The listing builds one solid part. Answer for the finished solid, in the listing's coordinates (mm). A direction names the side the tool comes from. Give positions to 0.01 mm unless a question says otherwise; leave off trailing zeros. Order: outer loops, then holes, each group sorted by start corner. A loop starts at its lowest first (then second) coordinate and runs counter-clockwise, first axis right, second up.
```python
from build123d import *

# Parameters (mm, degrees)
DIAM_TRE_DU_PER_AGE_4_0_4_1_D     = 4
DIAM_TRE_DU_PER_AGE_4_0_4_1_DEPTH = 5
DIAM_TRE_DU_PER_AGE_4_0_4_1_TIP   = 1.201721238
TROU_TARAUD_M41_D                 = 3.3
R_P_TITION_CIRCULAIRE1_COUNT      = 4
CHANFREIN1_SIZE                   = 0.5


with BuildPart() as part:
    # Esquisse1 → Révolution1 (revolve)
    with BuildSketch(Plane(origin=(0, 0, 0), x_dir=(0, 0, -1), z_dir=(1, 0, 0))):
        Polygon((-31, -3), (-31, 0), (-32.5, 0), (-32.5, 7), (-42, 7), (-42, -3), align=None)
    revolve(axis=Axis((0, 0, 0), (0, -1, 0)))

    # Diamètre du perçage Ø4.0 (4)1
    with Locations(Plane(origin=(0, 7, 0), x_dir=(1, 0, 0), z_dir=(0, 1, 0))):
        with Locations((0, 37), (0, -37)):
            Hole(DIAM_TRE_DU_PER_AGE_4_0_4_1_D / 2, depth=DIAM_TRE_DU_PER_AGE_4_0_4_1_DEPTH)
            with Locations((0, 0, -(DIAM_TRE_DU_PER_AGE_4_0_4_1_DEPTH + DIAM_TRE_DU_PER_AGE_4_0_4_1_TIP / 2))):  # 118° drill point
                Cone(0, DIAM_TRE_DU_PER_AGE_4_0_4_1_D / 2, DIAM_TRE_DU_PER_AGE_4_0_4_1_TIP, mode=Mode.SUBTRACT)

    # Trou taraudé M41 (through all)
    with Locations(Plane(origin=(0, 7, 0), x_dir=(1, 0, 0), z_dir=(0, 1, 0))):
        with Locations((-26.162950904, 26.162950904)):
            trou_taraud_m41 = Hole(TROU_TARAUD_M41_D / 2)

    # Répétition circulaire1: Trou taraudé M41 ×4 about axis
    r_p_tition_circulaire1_axis = Axis((0, 0, 0), (0, 1, 0))
    for i in range(1, R_P_TITION_CIRCULAIRE1_COUNT):
        add(trou_taraud_m41.rotate(r_p_tition_circulaire1_axis, i * 360 / R_P_TITION_CIRCULAIRE1_COUNT), mode=Mode.SUBTRACT)

    # Chanfrein1
    chanfrein1_edges = [part.edges().sort_by_distance(p)[0] for p in [
        (0, 7, -32.5),
    ]]
    chamfer(chanfrein1_edges, length=CHANFREIN1_SIZE)


solid = part.part
```
1) Given P1, Ø4, axis at x = 26.16, z = -26.16, coming from the +Y side; P2, Ø3, axis at x = -21, y = 2.5, coming from the +Z side; P3, Ø3, axis at y = 1.5, z = -18, coming from the +X side; P4, Ø5, axis at x = 13, y = 5.5, coming from the -Z side, each flat-ended and moving along its own axis, determine where each tip first touches the part or whether it passes through.
Geometry says:
P1: stops at y = 7
P2: stops at z = 37.2
P3: stops at x = 38.62
P4: stops at z = -40.67
2) A tool of negligible diameter and unlimited length cuts with its end or side. For faces 4 (the flat face through (12, 0, -29)), 5 (the cylindrical face through (-27.687, 1.93, -25.531)), from which of +Z, -Z, +X, -X, +Y, -Y can it reach the whole face along a straight path? Write none if from no direction.
Geometry says:
face 4: +Y
face 5: +Y, -Y
3) Find section A-A (z = 0). Write down the section's boundary in (x, y), then the cut area to 3 significant figures.
Geometry says:
outline: (-42, -3) - (-31, -3) - (-31, 0) - (-32.5, 0) - (-32.5, 6.5) - (-33, 7) - (-42, 7) - close; (31, -3) - (42, -3) - (42, 7) - (33, 7) - (32.5, 6.5) - (32.5, 0) - (31, 0) - close
area: 199 mm2
4) Straight lines are drawn through the part: probe 1 along Z at (x, y) = (0, 5.1); probe 2 along Z at (x, y) = (13, 6.25); probe 3 along X at (y, z) = (-0.75, -12). For each, find the intervals that lie inside material, in ascending order.
Geometry says:
probe 1: z = -42 to -39, -35 to -32.5, 32.5 to 35, 39 to 42
probe 2: z = -39.94 to -29.79, 29.79 to 39.94
probe 3: x = -40.25 to -28.58, 28.58 to 40.25
5) For a pull along X with two mould halves and no side action, classify faces 1 (the flat face through (31, 7, 13)), 2 (the cylindrical face through (27.687, 1.93, 25.531)), 3 (the cylindrical face through (-12.62, 1.93, 40.06)) as +X half, -X half, draft (parallel to the pull), parting line (faces both ways), or undercut.
Geometry says:
face 1: draft
face 2: undercut
face 3: parting line
